```python
from build123d import *

# Parameters (mm, degrees)
F2_DEPTH  = 9.525
F0_R      = 3.571875
F3_DEPTH  = 2.032
F3_FACE_R = 3.571875
F4_DEPTH  = 25.4


with BuildPart() as f2:
    # F1 (on Front) → F2 (new body, symmetric)
    with BuildSketch(Plane.XZ):
        with BuildLine():
            Line((-11.1125, 0), (11.1125, 0))
            ThreePointArc((11.1125, 0), (0, 11.1125), (-11.1125, 0))
        make_face()
    extrude(amount=F2_DEPTH, both=True)

    # F0 (on Top) → F3 (cut)
    with BuildSketch(Plane.XY):
        Polygon((5.55625, -3.207902), (5.55625, 3.207902), (0, 6.415805), (-5.55625, 3.207902), (-5.55625, -3.207902), (0, -6.415805), align=None)
        Circle(F0_R, mode=Mode.SUBTRACT)
    extrude(amount=F3_DEPTH, mode=Mode.SUBTRACT)

    # F3_face (on face) → F4 (cut)
    with BuildSketch(Plane(origin=(0, 0, 0), x_dir=(1, 0, 0), z_dir=(0, 0, -1))):
        Circle(F3_FACE_R)
    extrude(amount=-F4_DEPTH, mode=Mode.SUBTRACT)


solid = f2.part
```
Verification items for the finished model (mm, model axes). A direction names the side the tool comes from. Coordinates: 2 decimals unless noted, no trailing zeros. Loops run counter-clockwise (first coordinate to the right, second up) from the corner with the lowest first, then second, coordinate; pieces in that order, holes last. Notation, with made-up numbers: (-17.5, -15) - (15.5, -15) arc R17 ccw to (15.5, 1) - close; hole circle Ø9 at (46.5, 30). An arc over 180 degrees is marked (long way). Put each result on its own line as item: value.
Item 1: Section check D-D (y = 7.25). Enter the section's corners in (x, z) (1 decimal), then the cut area to 3 significant figures.
Conclusion:
outline: (-11.1, 0) - (11.1, 0) arc R11.1 ccw to start
area: 194 mm2
Item 2: Set-up check for faces 5 (the face through (3.4, -1.1, 6.5)), 6 (the face through (-2.739, 4.834, 1.002)): record each of +Z, -Z, +X, -X, +Y, -Y from which the full face is reachable in a straight line by a thin tool's end or side.
Conclusion:
face 5: +Z, -Z
face 6: -Z
Item 3: Draft check along Y on faces 1 (the face through (5.556, 0, 1)), 2 (the face through (0, -9.525, 4)), 3 (the face through (0, 9.525, 4)), 4 (the face through (-5.556, 0, 1)). Enter one of: pulls with the +Y half, pulls with the -Y half, needs draft (parallel to the pull), parting line crosses it, or undercut.
Conclusion:
face 1: undercut
face 2: pulls with the -Y half
face 3: pulls with the +Y half
face 4: undercut
Item 4: Section check C-C (z = 1.25). Enter the section's corners in (x, y) (3 decimals), then the cut area to 3 significant figures.
Conclusion:
outline: (-11.042, -9.525) - (11.042, -9.525) - (11.042, 9.525) - (-11.042, 9.525) - close; hole (-5.556, -3.208) - (0, -6.416) - (5.556, -3.208) - (5.556, 3.208) - (0, 6.416) - (-5.556, 3.208) - close
area: 314 mm2
Item 5: Section check A-A (x = -1.5). Enter the section's corners in (y, z) (3 decimals).
Conclusion:
outline: (-9.525, 0) - (-5.55, 0) - (-5.55, 2.032) - (-3.242, 2.032) - (-3.242, 11.011) - (-9.525, 11.011) - close; (3.242, 2.032) - (5.55, 2.032) - (5.55, 0) - (9.525, 0) - (9.525, 11.011) - (3.242, 11.011) - close
Item 6: Scan lines: line 1 along Y through (x, z) = (0, 8.5) (3 decimals); line 2 along Y through (x, z) = (-2.5, 10.5) (3 decimals); line 3 along X through (y, z) = (0, 8.75). Record each from-to range of solid material in increasing order.
Conclusion:
line 1: y = -9.525 to -3.572, 3.572 to 9.525
line 2: y = -9.525 to -2.551, 2.551 to 9.525
line 3: x = -6.85 to -3.57, 3.57 to 6.85
Item 7: Gauge pin test, flat ends, axial feed: pin 1 Ø4.5 at (x, y) = (0, 0) entering from +Z; pin 2 Ø0.6 at (y, z) = (-1.5, 0.5) entering from +X; pin 3 Ø2 at (y, z) = (-1, 1.5) entering from -X; pin 4 Ø3 at (x, y) = (4, 1) entering from -Z. Record the tip position at first contact, or that the pin passes through.
Conclusion:
pin 1: passes through
pin 2: stops at x = 11.11
pin 3: stops at x = -11.1
pin 4: stops at z = 2.03
Item 8: Section check B-B (y = 0). Enter the section's corners in (x, z) (1 decimal), then the cut area to 3 significant figures.
Conclusion:
outline: (-11.1, 0) - (-5.6, 0) - (-5.6, 2) - (-3.6, 2) - (-3.6, 10.5) arc R11.1 ccw to start; (3.6, 2) - (5.6, 2) - (5.6, 0) - (11.1, 0) arc R11.1 ccw to (3.6, 10.5) - close
area: 108 mm2
